Verification items for the finished model (mm, model axes). A direction names the side the tool comes from. Give positions to 0.01 mm unless a question says otherwise; leave off trailing zeros. One line per item, written item: value. Start each with the question number.
1. Gauge pin test, flat ends, axial feed: pin 1 (2 mm diameter, centred on x = 4.5, y = 9.5, fed in from +Z); pin 2 (1 mm diameter, centred on y = 2, z = -63.5, fed in from +X). Record the tip position at first contact, or that the pin passes through.
2. Mould release check, pull along Y, two halves, no side actions. Record for faces 1 (the flat face through (-5, 6, -52)), 2 (the flat face through (35, 12.5, -53)), 3 (the cylindrical face through (66.21, 4.42, -2.46)): pulls with the +Y half, pulls with the -Y half, needs draft (parallel to the pull), parting line crosses it, or undercut.
3. Scan lines: L1, parallel to X at y = 4.5, z = -57.5; L2, parallel to X at y = 1.75, z = -97.5. Record each from-to range of solid material in increasing order. Write a range as [from, to].
4. Access from +Z, -Z, +X, -X, +Y, -Y to the whole of each face (thin tool, end or side, straight path). Record for faces 4 (the flat face through (38, 6, -105)), 5 (the flat face through (70, 6, -5)).
from build123d import *

# Parameters (mm, degrees)
SKETCH1_W           = 80
SKETCH1_H           = 105
SKETCH1_W_2         = 5
BOSS_EXTRUDE1_DEPTH = 12.5
CUT_EXTRUDE1_DEPTH  = 5
FILLET1_R           = 5
FILLET2_R           = 5
FILLET3_R           = 2


with BuildPart() as part:
    # Sketch1 → Boss-Extrude1 (new body)
    with BuildSketch(Plane(origin=(0, 0, 0), x_dir=(1, 0, 0), z_dir=(0, 1, 0))):
        with Locations((40, 52.5)):
            Rectangle(SKETCH1_W, SKETCH1_H)
        with Locations((-2.5, 52.5)):
            Rectangle(SKETCH1_W_2, SKETCH1_H)
    extrude(amount=BOSS_EXTRUDE1_DEPTH)

    # Sketch2 → Cut-Extrude1 (cut)
    with BuildSketch(Plane.XY):
        with BuildLine():
            ThreePointArc((73, 2.895898034), (76.091650066, 3.44375696), (77.5, 6.25))
            Line((77.5, 6.25), (74, 6.25))
            Line((74, 6.25), (73, 6.25))
            Line((73, 6.25), (73, 2.895898034))
        make_face()
        with BuildLine():
            Line((74, 6.25), (77.5, 6.25))
            ThreePointArc((77.5, 6.25), (76.091650066, 9.05624304), (73, 9.604101966))
            Line((73, 9.604101966), (73, 6.25))
            Line((73, 6.25), (74, 6.25))
        make_face()
        with BuildLine():
            Line((73, 6.25), (73, 9.604101966))
            ThreePointArc((73, 9.604101966), (71.19375696, 8.341650066), (70.5, 6.25))
            Line((70.5, 6.25), (73, 6.25))
        make_face()
        with BuildLine():
            ThreePointArc((70.5, 6.25), (71.19375696, 4.158349934), (73, 2.895898034))
            Line((73, 2.895898034), (73, 6.25))
            Line((73, 6.25), (70.5, 6.25))
        make_face()
        with BuildLine():
            ThreePointArc((59.5, 5.25), (66.307499895, 4.402691993), (73, 2.895898034))
            ThreePointArc((73, 2.895898034), (71.19375696, 4.158349934), (70.5, 6.25))
            Line((70.5, 6.25), (59.5, 6.25))
            Line((59.5, 6.25), (58.5, 6.25))
            ThreePointArc((58.5, 6.25), (58.814539324, 5.564539324), (59.5, 5.25))
        make_face()
        with BuildLine():
            ThreePointArc((70.5, 6.25), (71.19375696, 8.341650066), (73, 9.604101966))
            ThreePointArc((73, 9.604101966), (66.311170081, 8.076260701), (59.5, 7.25))
            ThreePointArc((59.5, 7.25), (58.812768212, 6.937231788), (58.5, 6.25))
            Line((58.5, 6.25), (59.5, 6.25))
            Line((59.5, 6.25), (70.5, 6.25))
        make_face()
    extrude(amount=-CUT_EXTRUDE1_DEPTH, mode=Mode.SUBTRACT)

    # Fillet1
    fillet1_edges = [part.edges().sort_by_distance(p)[0] for p in [
        (80, 0, -52.5),
    ]]
    fillet(fillet1_edges, radius=FILLET1_R)

    # Fillet2
    fillet2_edges = [part.edges().sort_by_distance(p)[0] for p in [
        (80, 12.5, -52.5),
    ]]
    fillet(fillet2_edges, radius=FILLET2_R)

    # Fillet3
    fillet3_edges = [part.edges().sort_by_distance(p)[0] for p in [
        (-5, 12.5, -52.5),
        (-5, 0, -52.5),
    ]]
    fillet(fillet3_edges, radius=FILLET3_R)


solid = part.part
Results are:
1. pin 1: stops at z = 0
1. pin 2: stops at x = 79.33
2. face 1: needs draft
2. face 2: pulls with the +Y half
2. face 3: undercut
3. L1: x = [-5, 79.97]
3. L2: x = [-4.98, 78.8]
4. face 4: -Z, +X, -X, +Y, -Y
4. face 5: +Z
